from build123d import *

# Parameters (mm, degrees)
SKETCH1_R           = 3.45
SKETCH1_R_2         = 2.5
BOSS_EXTRUDE1_DEPTH = 4.4
SKETCH1_3_W         = 15
SKETCH1_3_H         = 10
SKETCH1_3_R         = 3.45
BOSS_EXTRUDE2_DEPTH = 1.6
FILLET1_R           = 2


with BuildPart() as part:
    # Sketch1 → Boss-Extrude1 (new body)
    with BuildSketch(Plane.XY):
        Circle(SKETCH1_R)
        Circle(SKETCH1_R_2, mode=Mode.SUBTRACT)
    extrude(amount=BOSS_EXTRUDE1_DEPTH)

    # Sketch1<3> → Boss-Extrude2 (add)
    with BuildSketch(Plane.XY):
        Rectangle(SKETCH1_3_W, SKETCH1_3_H)
        Circle(SKETCH1_3_R, mode=Mode.SUBTRACT)
    extrude(amount=BOSS_EXTRUDE2_DEPTH)

    # Fillet1
    # the kernel refuses this fillet: 2 mm, written as the material it takes off along each edge
    with BuildSketch(Plane(origin=(0, 0, 4.4), x_dir=(1, 0, 0), z_dir=(0, -1, 0))) as fillet1_piece_1:
        with BuildLine():
            CenterArc((1.45, -1.702204453), FILLET1_R, 0, 58.331756746)
            Line((2.5, 0), (2.521, 0.034044089))
            ThreePointArc((2.521, 0.034044089), (2.975, 0.04), (3.45, 0.04))
            Line((3.45, 0.04), (3.49, 0))
            Line((3.49, 0), (3.49, -1.702204453))
            Line((3.49, -1.702204453), (3.45, -1.702204453))
        make_face()
    revolve(axis=Axis((0, 0, 4.4), (0, 0, 1)), mode=Mode.SUBTRACT)


solid = part.part
Source: CAD feature listing. Evaluate the final solid. Frame: model axes, mm. A direction names the side the tool comes from. Coordinates: 2 decimals unless noted, no trailing zeros. Write each loop counter-clockwise with the first axis right and the second up, starting at its lowest first coordinate (ties: lowest second). Pieces come first, ordered by that corner, then holes. Notation, with made-up numbers: M 76,70 L 88,70 A18 cw 88,75 Z; hole C 37,41.5 d7. An arc over 180 degrees is marked long. Use a Markdown table: item, result.
1) Section C-C, the plane x = 5.75. Output: boundary loops of the cut face in (y, z).
Conclusion:
| item | result |
|---|---|
| outline | M -5,0 L 5,0 L 5,1.6 L -5,1.6 Z |
2) First-contact query: pin 1 Ø1.5 at (x, y) = (-6, -2.5) entering from +Z; pin 2 Ø1.5 at (x, y) = (-2.5, 0) entering from -Z; pin 3 Ø1 at (y, z) = (1.5, 3.5) entering from +X; pin 4 Ø2 at (x, y) = (-3.5, 2) entering from +Z. Flat tips, straight axial feed; report the tip coordinate or a pass-through.
Conclusion:
| item | result |
|---|---|
| pin 1 | stops at z = 1.6 |
| pin 2 | stops at z = 0 |
| pin 3 | stops at x = 3.2 |
| pin 4 | stops at z = 3.92 |
3) Section B-B, the plane y = -4. Output: boundary loops of the cut face in (x, z), then the cut area to 3 significant figures.
Conclusion:
| item | result |
|---|---|
| outline | M -7.5,0 L 7.5,0 L 7.5,1.6 L -7.5,1.6 Z |
| area | 24.0 mm^2 |
4) Ray query, L1, parallel to Y at x = 0, z = 0.95; L2, parallel to Z at x = -4.75, y = -0.25; L3, parallel to Y at x = 0, z = 2.25. Return the intervals inside material, ascending.
Conclusion:
| item | result |
|---|---|
| L1 | y = -5 to -2.5, 2.5 to 5 |
| L2 | z = 0 to 1.6 |
| L3 | y = -3.45 to -2.5, 2.5 to 3.45 |
5) Mould query, pull axis X, two halves, no side actions, for faces 3 (the cylindrical face through (-0.54, -2.44, 2.17)), 4 (the flat face through (-7.5, 0, 1)), 5 (the flat face through (-2, 2, 0)). Classes: pulls with the +X half, pulls with the -X half, needs draft (parallel to the pull), parting line crosses it, or undercut.
Conclusion:
| item | result |
|---|---|
| face 3 | undercut |
| face 4 | pulls with the -X half |
| face 5 | needs draft |
6) Section A-A, the plane z = 1.4. Output: boundary loops of the cut face in (x, y), then the cut area to 3 significant figures.
Conclusion:
| item | result |
|---|---|
| outline | M -7.5,-5 L 7.5,-5 L 7.5,5 L -7.5,5 Z; hole C 0,0 d5 |
| area | 130 mm^2 |
7) Reachability of faces 1 (the cylindrical face through (-0.45, 3.42, 2.14)), 2 (the flat face through (0, -5, 1)) from +Z, -Z, +X, -X, +Y, -Y: full face, straight path, thin tool, end or side. Return the list, or none.
Conclusion:
| item | result |
|---|---|
| face 1 | +Z |
| face 2 | +Z, -Z, +X, -X, -Y |
